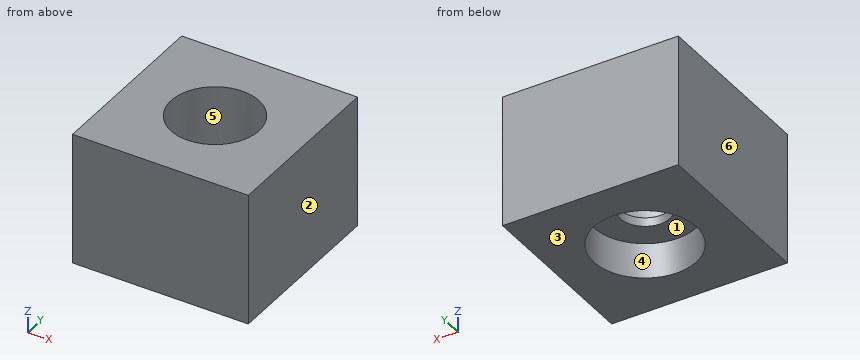
```python
from build123d import *

# Parameters (mm, degrees)
ESQUISSE1_W                                        = 12
ESQUISSE1_H                                        = 12
ESQUISSE1_R                                        = 3
BOSS_EXTRU_1_DEPTH                                 = 6
ESQUISSE2_W                                        = 12
ESQUISSE2_H                                        = 12
BOSS_EXTRU_2_DEPTH                                 = 3
CHAMBRAGE_POUR_VIS_T_TE_RONDE_BOMB_E_M_D           = 3.4
CHAMBRAGE_POUR_VIS_T_TE_RONDE_BOMB_E_M_DEPTH       = 6.35
CHAMBRAGE_POUR_VIS_T_TE_RONDE_BOMB_E_M_CBORE_D     = 7
CHAMBRAGE_POUR_VIS_T_TE_RONDE_BOMB_E_M_CBORE_DEPTH = 2.4


with BuildPart() as part:
    # Esquisse1 → Boss.-Extru.1 (new body)
    with BuildSketch(Plane.XY):
        Rectangle(ESQUISSE1_W, ESQUISSE1_H)
        Circle(ESQUISSE1_R, mode=Mode.SUBTRACT)
    extrude(amount=BOSS_EXTRU_1_DEPTH)

    # Esquisse2 → Boss.-Extru.2 (add)
    with BuildSketch(Plane(origin=(0, 0, 0), x_dir=(-1, 0, 0), z_dir=(0, 0, -1))):
        Rectangle(ESQUISSE2_W, ESQUISSE2_H)
    extrude(amount=BOSS_EXTRU_2_DEPTH)

    # Chambrage pour vis à tête ronde bombée M31
    with Locations(Plane(origin=(0, 0, -3), x_dir=(-1, 0, 0), z_dir=(0, 0, -1))):
        with Locations((0, 0)):
            CounterBoreHole(CHAMBRAGE_POUR_VIS_T_TE_RONDE_BOMB_E_M_D / 2, CHAMBRAGE_POUR_VIS_T_TE_RONDE_BOMB_E_M_CBORE_D / 2, CHAMBRAGE_POUR_VIS_T_TE_RONDE_BOMB_E_M_CBORE_DEPTH, depth=CHAMBRAGE_POUR_VIS_T_TE_RONDE_BOMB_E_M_DEPTH)


solid = part.part
```
The listing builds one solid part. Answer for the finished solid, in the listing's coordinates (mm). Face numbers are marked on the shaded views. A direction names the side the tool comes from. Give positions to 0.01 mm unless a question says otherwise; leave off trailing zeros. Order: outer loops, then holes, each group sorted by start corner. A loop starts at its lowest first (then second) coordinate and runs counter-clockwise, first axis right, second up. Notation, with made-up numbers: (-29, 26) -> (6, 26) arc R33 ccw to (6, 64) -> close; hole circle Ø6 at (28, -31). An arc over 180 degrees is marked (long way). Answer as CSV lines item,"result". Start each with the question number.
Q1. Find the intervals of material crossed by L1, parallel to Y at x = 0, z = 1.4; L2, parallel to Y at x = -1.5, z = 2.5; L3, parallel to Z at x = -1.75, y = 0.5, in increasing order.
Q2. A cutting plane is placed at D-D (y = 2.75). Determine the outline of the cut face in (x, z), then the cut area to 3 significant figures.
Q3. Which of the six approach directions +Z, -Z, +X, -X, +Y, -Y give full straight-line access (tool end or side, diameter ignored) to the marked faces 4, 5 and 6?
Q4. Given pin 1 (2 mm diameter, centred on x = 1.5, y = 1.5, fed in from -Z); pin 2 (4.5 mm diameter, centred on x = 0, y = 0, fed in from +Z); pin 3 (7 mm diameter, centred on x = 0, y = 0, fed in from +Z); pin 4 (1.8 mm diameter, centred on x = -0.5, y = 0.5, fed in from +Z), each flat-ended and moving along its own axis, determine where each tip first touches the part or whether it passes through.
Q5. Determine the mould class of the marked faces 1, 2 and 3 for opening direction X: pulls with the +X half, pulls with the -X half, needs draft (parallel to the pull), parting line crosses it, or undercut.
Q6. A cutting plane is placed at A-A (y = 0). Determine the outline of the cut face in (x, z), then the cut area to 3 significant figures.
Q7. A cutting plane is placed at C-C (z = 3.5). Determine the outline of the cut face in (x, y).
Results found:
1,L1,"-6 to -3, 3 to 6"
1,L2,"-6 to -2.6, 2.6 to 6"
1,L3,"-0.6 to 0"
2,outline,"(-6, -3) -> (-2.17, -3) -> (-2.17, -0.6) -> (2.17, -0.6) -> (2.17, -3) -> (6, -3) -> (6, 6) -> (1.2, 6) -> (1.2, 0) -> (-1.2, 0) -> (-1.2, 6) -> (-6, 6) -> close"
2,area,"83.2 mm2"
3,face 4,"-Z"
3,face 5,"+Z"
3,face 6,"+Z, -Z, -X, +Y, -Y"
4,pin 1,"z = -0.6"
4,pin 2,"z = 0"
4,pin 3,"z = 6"
4,pin 4,"through"
5,face 1,"undercut"
5,face 2,"pulls with the +X half"
5,face 3,"needs draft"
6,outline,"(-6, -3) -> (-3.5, -3) -> (-3.5, -0.6) -> (-1.7, -0.6) -> (-1.7, 0) -> (-3, 0) -> (-3, 6) -> (-6, 6) -> close; (1.7, -0.6) -> (3.5, -0.6) -> (3.5, -3) -> (6, -3) -> (6, 6) -> (3, 6) -> (3, 0) -> (1.7, 0) -> close"
6,area,"53.2 mm2"
7,outline,"(-6, -6) -> (6, -6) -> (6, 6) -> (-6, 6) -> close; hole circle Ø6 at (0, 0)"
